Answer from the drawing. Dimensions are ordinates in mm from the lowest x, y and z of the part. A direction names the side the tool comes from. Give positions to 0.01 mm unless a question says otherwise; leave off trailing zeros. Order: outer loops, then holes, each group sorted by start corner. A loop starts at its lowest first (then second) coordinate and runs counter-clockwise, first axis right, second up.
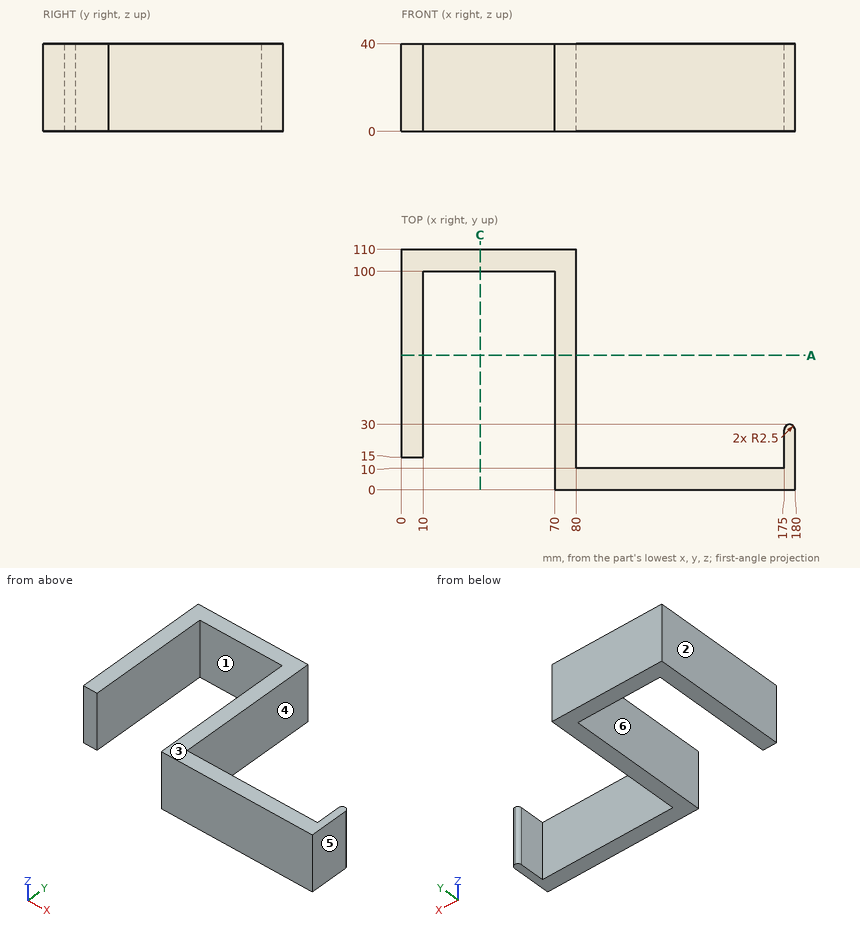
1. The mould has two halves that part along X. Classify the marked faces 1, 2 and 3: pulls with the +X half, pulls with the -X half, needs draft (parallel to the pull), parting line crosses it, or undercut.
Findings below:
face 1: undercut
face 2: pulls with the -X half
face 3: needs draft
2. The part is cut by section C-C (x = 36). Write down the section's boundary in (y, z), then the cut area to 3 significant figures.
Findings below:
outline: (100, 0) - (110, 0) - (110, 40) - (100, 40) - close
area: 400 mm2
3. The part is cut by section A-A (y = 61.5). Write down the section's boundary in (x, z).
Findings below:
outline: (0, 0) - (10, 0) - (10, 40) - (0, 40) - close; (70, 0) - (80, 0) - (80, 40) - (70, 40) - close
4. Straight lines are drawn through the part: probe 1 along X at (y, z) = (20, 2); probe 2 along X at (y, z) = (14, 16.5); probe 3 along X at (y, z) = (96, 24.5). For each, find the intervals that lie inside material, in ascending order.
Findings below:
probe 1: x = 0 to 10, 70 to 80, 175 to 180
probe 2: x = 70 to 80, 175 to 180
probe 3: x = 0 to 10, 70 to 80
5. Which of the six approach directions +Z, -Z, +X, -X, +Y, -Y give full straight-line access (tool end or side, diameter ignored) to the marked faces 4, 5 and 6?
Findings below:
face 4: +Z, -Z, +Y
face 5: +Z, -Z, +X, +Y, -Y
face 6: +Z, -Z, -Y
6. Given P1, Ø8, axis at x = 4.5, z = 18.5, coming from the -Y side; P2, Ø4, axis at x = 96, z = 12, coming from the +Y side; P3, Ø20, axis at x = 40, z = 10.5, coming from the -Y side, each flat-ended and moving along its own axis, determine where each tip first touches the part or whether it passes through.
Findings below:
P1: stops at y = 15
P2: stops at y = 10
P3: stops at y = 100
